Can you work these out from the drawing? Everything is in mm from the part's minimum corner. A direction names the side the tool comes from. Coordinates: 2 decimals unless noted, no trailing zeros. Loops run counter-clockwise (first coordinate to the right, second up) from the corner with the lowest first, then second, coordinate; pieces in that order, holes last. Notation, with made-up numbers: (87.5, 59) -> (108.5, 59) arc R7 ccw to (108.5, 72) -> close; hole circle Ø9 at (-29, -38). An arc over 180 degrees is marked (long way). One line per question, with ' | ' between items.
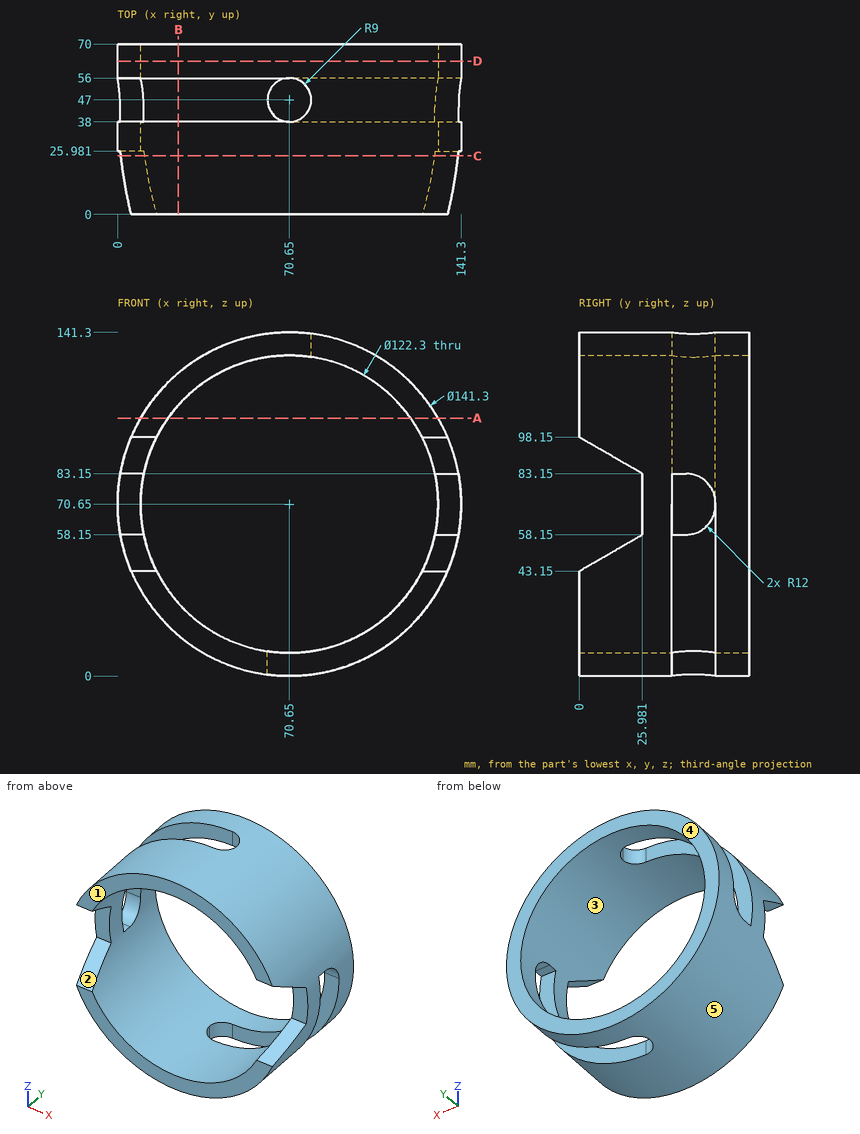
Q1. Imagine slicing it at B-B on x = 25. Write out the boundary of the cut face in (y, z).
Values follow:
outline: (0, 16.73) -> (70, 16.73) -> (70, 29.96) -> (0, 29.96) -> close; (0, 111.34) -> (38, 111.34) -> (38, 124.57) -> (0, 124.57) -> close; (56, 111.34) -> (70, 111.34) -> (70, 124.57) -> (56, 124.57) -> close
Q2. Imagine slicing it at C-C on y = 24. Write out the boundary of the cut face in (x, z), plus the area to 3 significant figures.
Values follow:
outline: (1.33, 57.01) arc R70.65 ccw to (139.97, 57.01) -> (130.26, 57.01) arc R61.15 cw to (11.04, 57.01) -> close; (1.33, 84.29) -> (11.04, 84.29) arc R61.15 cw to (130.26, 84.29) -> (139.97, 84.29) arc R70.65 ccw to start | area: 3,410 mm2
Q3. Imagine slicing it at A-A on z = 106. Write out the boundary of the cut face in (x, y).
Values follow:
outline: (9.48, 0) -> (20.75, 0) -> (20.75, 38) -> (9.48, 38) -> close; (9.48, 56) -> (20.75, 56) -> (20.75, 70) -> (9.48, 70) -> close; (120.55, 0) -> (131.82, 0) -> (131.82, 70) -> (120.55, 70) -> close
Q4. Please list where these lines run through material, in increasing order: L1, parallel to Z at x = 70, y = 33; L2, parallel to X at y = 33.5, z = 64. Write a range as [from, to].
Values follow:
L1: z = [0, 9.5], [131.8, 141.3] | L2: x = [0.31, 9.86], [131.44, 140.99]
Q5. For the marked faces 1 and 2, which set-ups out of +Z, -Z, +X, -X, +Y, -Y let a thin tool reach every point of the face, with its end or its side?
Values follow:
face 1: +Z, -Z, +X, -X, -Y | face 2: +X, -X, -Y
Q6. For pin 1 (5.5 mm diameter, centred on x = 137, z = 73.5, fed in from -Y); pin 2 (10 mm diameter, centred on y = 24.5, z = 87.5, fed in from +X); pin 3 (1.5 mm diameter, centred on x = 113, y = 19, fed in from -Z), each with a flat end and sliding along its axis, tell me the tip position at first contact or that it passes through.
Values follow:
pin 1: stops at y = 25.98 | pin 2: stops at x = 140.26 | pin 3: stops at z = 13.55
Q7. We'd pull the mould along X, two halves only. Please class the marked faces 3, 4 and 5: released by +X, released by -X, zero draft, split by the parting line, or undercut.
Values follow:
face 3: undercut | face 4: zero draft | face 5: split by the parting line
Q8. Imagine slicing it at D-D on y = 63. Write out the boundary of the cut face in (x, z), plus the area to 3 significant figures.
Values follow:
outline: circle Ø141.3 at (70.65, 70.65); hole circle Ø122.3 at (70.65, 70.65) | area: 3,930 mm2
